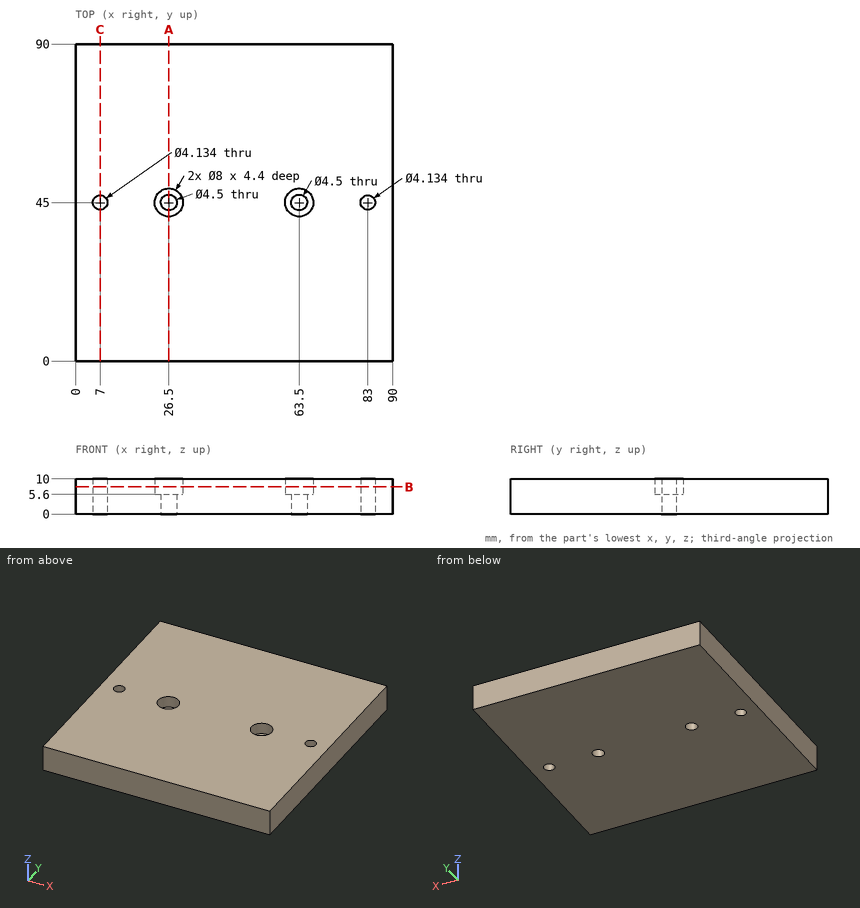
Drawing for the job (mm, zero at the part's lowest x, y, z). Round coordinates to 2 decimals unless told otherwise and drop trailing zeros. Loops run counter-clockwise (first coordinate to the right, second up) from the corner with the lowest first, then second, coordinate; pieces in that order, holes last. Notation, with made-up numbers: (5.25, -7.75) -> (27.25, -7.75) arc R22 ccw to (27.25, 22.25) -> close; hole circle Ø2 at (0, -16). An arc over 180 degrees is marked (long way). Use one line per item in the form item = value. Start each with the question number.
Item 1: Drill centre lines: line 1 along X through (y, z) = (45, 8.85); line 2 along Y through (x, z) = (63.5, 3.05); line 3 along X through (y, z) = (45, 3.95). Where is each one in solid material? Low to high.
Item 2: Band-saw the part on C-C (x = 7). List the corners of the cut face in (y, z), plus the area to 3 significant figures.
Item 3: Band-saw the part on A-A (x = 26.5). List the corners of the cut face in (y, z), plus the area to 3 significant figures.
Item 4: Drop flat-ended pins along their axis: pin 1 Ø5 at (x, y) = (26.5, 45) entering from -Z; pin 2 Ø3.5 at (x, y) = (83, 45) entering from -Z; pin 3 Ø2.5 at (x, y) = (26, 46.5) entering from +Z. Give the stop position or say it passes through.
Item 5: Band-saw the part on B-B (z = 7.75). List the corners of the cut face in (x, y).
Data:
q1.line_1 = 0 to 4.93, 9.07 to 22.5, 30.5 to 59.5, 67.5 to 80.93, 85.07 to 90
q1.line_2 = 0 to 42.75, 47.25 to 90
q1.line_3 = 0 to 4.93, 9.07 to 24.25, 28.75 to 61.25, 65.75 to 80.93, 85.07 to 90
q2.outline = (0, 0) -> (42.93, 0) -> (42.93, 10) -> (0, 10) -> close; (47.07, 0) -> (90, 0) -> (90, 10) -> (47.07, 10) -> close
q2.area = 859 mm^2
q3.outline = (0, 0) -> (42.75, 0) -> (42.75, 5.6) -> (41, 5.6) -> (41, 10) -> (0, 10) -> close; (47.25, 0) -> (90, 0) -> (90, 10) -> (49, 10) -> (49, 5.6) -> (47.25, 5.6) -> close
q3.area = 840 mm^2
q4.pin_1 = 0
q4.pin_2 = through
q4.pin_3 = 5.6
q5.outline = (0, 0) -> (90, 0) -> (90, 90) -> (0, 90) -> close; hole circle Ø4.13 at (7, 45); hole circle Ø8 at (26.5, 45); hole circle Ø8 at (63.5, 45); hole circle Ø4.13 at (83, 45)
